Design review of the part built by this model. Coordinates are the model's own, in mm. A direction names the side the tool comes from. Round coordinates to 2 decimals unless told otherwise and drop trailing zeros. Write each loop counter-clockwise with the first axis right and the second up, starting at its lowest first coordinate (ties: lowest second). Pieces come first, ordered by that corner, then holes. Notation, with made-up numbers: M 21,78 L 50,78 A19 ccw 50,96 Z; hole C 6,52 d6. An arc over 180 degrees is marked long. Use CSV: the item, a comma, the result in double quotes.
from build123d import *

# Parameters (mm, degrees)
F0_W     = 107.738086
F0_H     = 70.393864
F1_DEPTH = 25.4
F2_R     = 24.783806
F3_DEPTH = 25.4
F4_R     = 18.605806
F5_DEPTH = 76.2


with BuildPart() as f1:
    # F0 (on Front) → F1 (new body)
    with BuildSketch(Plane.XZ):
        with Locations((0.186719, 2.147293)):
            Rectangle(F0_W, F0_H)
    extrude(amount=F1_DEPTH)

    # F2 (on face) → F3 (join)
    with BuildSketch(Plane.XZ.offset(25.4)):
        Circle(F2_R)
    extrude(amount=F3_DEPTH)

    # F4 (on face) → F5 (cut)
    with BuildSketch(Plane.XZ.offset(50.8)):
        Circle(F4_R)
    extrude(amount=-F5_DEPTH, mode=Mode.SUBTRACT)


solid = f1.part
1) Wall thickness on line 1 along Z through (x, y) = (0, -37); line 2 along X through (y, z) = (-30, -1); line 3 along Z through (x, y) = (0, -17.5): over which ranges is each line inside the solid? List them lowest first. Write a range as [from, to].
Answers:
line 1,"[-24.78, -18.61], [18.61, 24.78]"
line 2,"[-24.76, -18.58], [18.58, 24.76]"
line 3,"[-33.05, -18.61], [18.61, 37.34]"
2) Add section D-D on x = -27. Write out the cut boundary in (y, z).
Answers:
outline,"M -25.4,-33.05 L 0,-33.05 L 0,37.34 L -25.4,37.34 Z"
3) Machinability: for faces 1 (the face through (-1, -13, 37.344)), 2 (the face through (-1, -25.4, 26)), which of the approach directions +Z, -Z, +X, -X, +Y, -Y give a long, thin tool a straight path to every point of the face, cutting with its end or side? Answer none if there is none.
Answers:
face 1,"+Z, +X, -X, +Y, -Y"
face 2,"-Y"
4) Add section C-C on y = -23. Write out the cut boundary in (x, z), then the cut area to 3 significant figures.
Answers:
outline,"M -53.68,-33.05 L 54.06,-33.05 L 54.06,37.34 L -53.68,37.34 Z; hole C 0,0 d37.21"
area,"6,500 mm²"
5) For pin 1 Ø10 at (x, z) = (-42, 0) entering from -Y; pin 2 Ø6 at (y, z) = (-36, 17) entering from -X, all flat-tipped, find the tip position at first contact; note any pin that passes through.
Answers:
pin 1,"y = -25.4"
pin 2,"x = -20.45"
6) Add section B-B on x = 0. Write out the cut boundary in (y, z).
Answers:
outline,"M -50.8,-24.78 L -25.4,-24.78 L -25.4,-33.05 L 0,-33.05 L 0,-18.61 L -50.8,-18.61 Z; M -50.8,18.61 L 0,18.61 L 0,37.34 L -25.4,37.34 L -25.4,24.78 L -50.8,24.78 Z"
7) Add section A-A on z = 0. Write out the cut boundary in (x, y).
Answers:
outline,"M -53.68,-25.4 L -24.78,-25.4 L -24.78,-50.8 L -18.61,-50.8 L -18.61,0 L -53.68,0 Z; M 18.61,-50.8 L 24.78,-50.8 L 24.78,-25.4 L 54.06,-25.4 L 54.06,0 L 18.61,0 Z"
